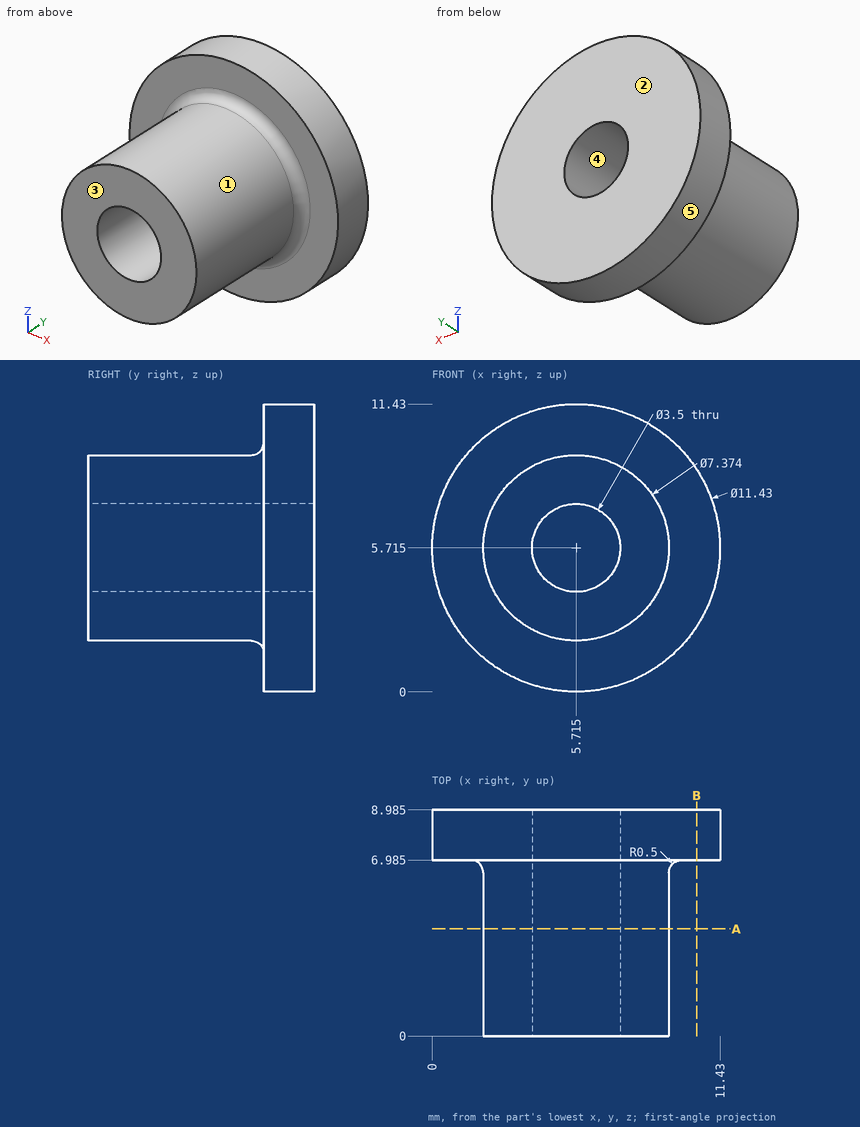
Answer from the drawing. Dimensions are ordinates in mm from the lowest x, y and z of the part. A direction names the side the tool comes from. Give positions to 0.01 mm unless a question says otherwise; leave off trailing zeros. Loops run counter-clockwise (first coordinate to the right, second up) from the corner with the lowest first, then second, coordinate; pieces in that order, holes last. Notation, with made-up numbers: (77.25, 13) -> (121.25, 13) arc R19 ccw to (121.25, 39) -> close; hole circle Ø8 at (47.25, -10). An arc over 180 degrees is marked (long way). Answer as CSV lines item,"result".
Item 1: Determine the mould class of the marked faces 3, 4 and 5 for opening direction Z: +Z half, -Z half, draft (parallel to the pull), parting line (faces both ways), or undercut.
Returned:
face 3,"draft"
face 4,"undercut"
face 5,"parting line"
Item 2: Find section B-B on x = 10.5. Give the vertices of the cut face in (y, z) (3 decimals).
Returned:
outline,"(6.985, 2.59) -> (8.985, 2.59) -> (8.985, 8.84) -> (6.985, 8.84) -> close"
Item 3: For the marked faces 1 and 2, determine the directions among +Z, -Z, +X, -X, +Y, -Y from which every point of the face is accessible in a straight line to the end or side of a thin tool.
Returned:
face 1,"-Y"
face 2,"+Z, -Z, +X, -X, +Y"
Item 4: Each of these flat-tipped pins is pushed along its axis until it touches: pin 1 (4 mm diameter, centred on x = 2.5, z = 9.5, fed in from -Y); pin 2 (3 mm diameter, centred on x = 9.5, y = 6.5, fed in from -Z); pin 3 (5 mm diameter, centred on x = 9, y = 2, fed in from +Z); pin 4 (4 mm diameter, centred on y = 3.5, z = 5.5, fed in from +X). Where does it stop, or does it pass through?
Returned:
pin 1,"stops at y = 0"
pin 2,"stops at z = 0.51"
pin 3,"stops at z = 9.32"
pin 4,"stops at x = 9.4"
Item 5: Consider line 1 (X direction, y = 7.25, z = 5.75); line 2 (Z direction, x = 6.5, y = 4.75); line 3 (Y direction, x = 7.25, z = 1) (3 decimals). Determine where each line is inside the solid, lowest interval first. Write a range as [from, to].
Returned:
line 1,"x = [0, 3.97], [7.46, 11.43]"
line 2,"z = [2.11, 4.15], [7.28, 9.32]"
line 3,"y = [6.985, 8.985]"
Item 6: Find section A-A on y = 4.25. Give the vertices of the cut face in (x, z) (3 decimals), plus the area to 3 significant figures.
Returned:
outline,"circle Ø7.374 at (5.715, 5.715); hole circle Ø3.5 at (5.715, 5.715)"
area,"33.1 mm²"
